Work out the finished part from the listing and answer in its coordinate system (mm). Face numbers are marked on the shaded views. A direction names the side the tool comes from. Coordinates: 2 decimals unless noted, no trailing zeros. Order: outer loops, then holes, each group sorted by start corner. A loop starts at its lowest first (then second) coordinate and runs counter-clockwise, first axis right, second up.
1. The part is cut by section B-B, the plane z = -4. Give the vertices of the cut face in (x, y).
2. Flat-ended cylindrical pins translate along their axes: pin 1 Ø1 at (x, y) = (-2.5, 8.5) entering from +Z; pin 2 Ø4.5 at (x, z) = (0, -25) entering from -Y (3 decimals); pin 3 Ø1 at (x, y) = (-3.5, 17.5) entering from +Z; pin 4 Ø5 at (x, y) = (-4, 8.5) entering from -Z. Find the tip coordinate at first contact, or state that the pin passes through.
3. The part is cut by section D-D, the plane y = 3.5. Give the vertices of the cut face in (x, z), then the cut area to 3 significant figures.
4. The part is cut by section A-A, the plane y = 10. Give the vertices of the cut face in (x, z).
5. The part is cut by section C-C, the plane x = 1.75. Count the separate pieces of the cut face and the enclosed holes in it, then the cut area to 3 significant figures.
6. A tool of negligible diameter and unlimited length cuts with its end or side. For the marked faces 5, 6 and 7, from which of +Z, -Z, +X, -X, +Y, -Y can it reach the whole face along a straight path? Write none if from no direction.
7. Determine the mould class of the marked faces 1, 2, 3 and 4 for opening direction Y: +Y half, -Y half, draft (parallel to the pull), parting line (faces both ways), or undercut.
8. Find the intervals of material crossed by probe 1 along Y at (x, z) = (0.25, 12); probe 2 along Z at (x, y) = (0, 9.5); probe 3 along X at (y, z) = (18.8, 25), in increasing order.
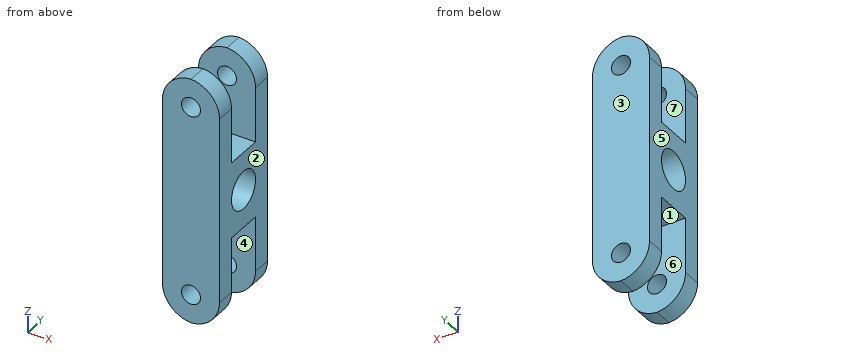
```python
from build123d import *

# Parameters (mm, degrees)
SKETCH1_W           = 15
SKETCH1_H           = 65
BOSS_EXTRUDE1_DEPTH = 20
SKETCH2_R           = 2.5
CUT_EXTRUDE1_DEPTH  = 20
SKETCH6_R           = 5
CUT_EXTRUDE3_DEPTH  = 15
SKETCH7_W           = 22.5
SKETCH7_H           = 5
SKETCH7_H_2         = 10
CUT_EXTRUDE4_DEPTH  = 15
FILLET3_R           = 8


with BuildPart() as part:
    # Sketch1 → Boss-Extrude1 (new body)
    with BuildSketch(Plane(origin=(0, 0, 0), x_dir=(1, 0, 0), z_dir=(0, 1, 0))):
        Rectangle(SKETCH1_W, SKETCH1_H)
    extrude(amount=BOSS_EXTRUDE1_DEPTH)

    # Sketch2 → Cut-Extrude1 (cut)
    with BuildSketch(Plane(origin=(0, 20, 0), x_dir=(1, 0, 0), z_dir=(0, 1, 0))):
        with Locations(Location((0, 25, 0), (0, 0, 270))):
            Circle(SKETCH2_R)
        with Locations(Location((0, -25, 0), (0, 0, 90))):
            Circle(SKETCH2_R)
    extrude(amount=-CUT_EXTRUDE1_DEPTH, mode=Mode.SUBTRACT)

    # Sketch6 → Cut-Extrude3 (cut)
    with BuildSketch(Plane(origin=(7.5, 0, 0), x_dir=(0, 0, -1), z_dir=(1, 0, 0))):
        with Locations((0, 10)):
            Circle(SKETCH6_R)
    extrude(amount=-CUT_EXTRUDE3_DEPTH, mode=Mode.SUBTRACT)

    # Sketch7 → Cut-Extrude4 (cut)
    with BuildSketch(Plane(origin=(7.5, 0, 0), x_dir=(0, 0, -1), z_dir=(1, 0, 0))):
        with Locations((-21.25, 12.5)):
            Rectangle(SKETCH7_W, SKETCH7_H)
        with Locations((-21.25, 7.5)):
            Rectangle(SKETCH7_W, SKETCH7_H)
        with Locations((21.25, 10)):
            Rectangle(SKETCH7_W, SKETCH7_H_2)
    extrude(amount=-CUT_EXTRUDE4_DEPTH, mode=Mode.SUBTRACT)

    # Fillet3
    # the kernel refuses this fillet: 8 mm, written as the material it takes off along each edge
    with BuildSketch(Plane(origin=(-7.5, -20, 32.5), x_dir=(1, 0, 0), z_dir=(0, 1, 0)), Plane(origin=(-7.5, -20, -32.5), x_dir=(0, 0, 1), z_dir=(0, 1, 0)), Plane(origin=(-7.5, -5, -32.5), x_dir=(0, 0, 1), z_dir=(0, 1, 0)), Plane(origin=(7.5, -5, 32.5), x_dir=(0, 0, -1), z_dir=(0, 1, 0))) as fillet3_piece_1:
        with BuildLine():
            CenterArc((FILLET3_R, FILLET3_R), FILLET3_R, 180, 90)
            Line((0, FILLET3_R), (0, 0))
            Line((0, 0), (FILLET3_R, 0))
        make_face()
    extrude(amount=45, mode=Mode.SUBTRACT)
    with BuildSketch(Plane(origin=(7.5, -20, 32.5), x_dir=(-1, 0, 0), z_dir=(0, 1, 0)), Plane(origin=(7.5, -20, -32.5), x_dir=(0, 0, 1), z_dir=(0, 1, 0)), Plane(origin=(7.5, -5, -32.5), x_dir=(0, 0, 1), z_dir=(0, 1, 0)), Plane(origin=(-7.5, -5, 32.5), x_dir=(0, 0, -1), z_dir=(0, 1, 0))) as fillet3_piece_2:
        with BuildLine():
            CenterArc((FILLET3_R, -FILLET3_R), FILLET3_R, 90, 90)
            Line((0, -FILLET3_R), (0, 0))
            Line((0, 0), (FILLET3_R, 0))
        make_face()
    extrude(amount=45, mode=Mode.SUBTRACT)


solid = part.part
```
Geometry says:
1. outline: (-7.5, 0) - (7.5, 0) - (7.5, 7) - (-7.5, 7) - close; (-7.5, 13) - (7.5, 13) - (7.5, 20) - (-7.5, 20) - close
2. pin 1: stops at z = 10
2. pin 2: passes through
2. pin 3: stops at z = 31.69
2. pin 4: stops at z = -10
3. outline: (-7.5, -24.5) arc R8 ccw to (0, -32.48) arc R8 ccw to (7.5, -24.5) - (7.5, 24.5) arc R8 ccw to (0, 32.48) arc R8 ccw to (-7.5, 24.5) - close; hole circle Ø5 at (0, -25); hole circle Ø5 at (0, 25)
3. area: 881 mm2
4. outline: (-7.5, -10) - (7.5, -10) - (7.5, -5) - (-7.5, -5) - close; (-7.5, 5) - (7.5, 5) - (7.5, 10) - (-7.5, 10) - close
5. separate pieces: 5
5. enclosed holes: 1
5. area: 694 mm2
6. face 5: +Z, -Z, -X, +Y, -Y
6. face 6: -Z, +X, -X
6. face 7: +Z, +X, -X
7. face 1: undercut
7. face 2: draft
7. face 3: +Y half
7. face 4: undercut
8. probe 1: y = 0 to 5, 15 to 20
8. probe 2: z = -10 to -4.97, 4.97 to 10
8. probe 3: x = -7.48 to -2.5, 2.5 to 7.48
